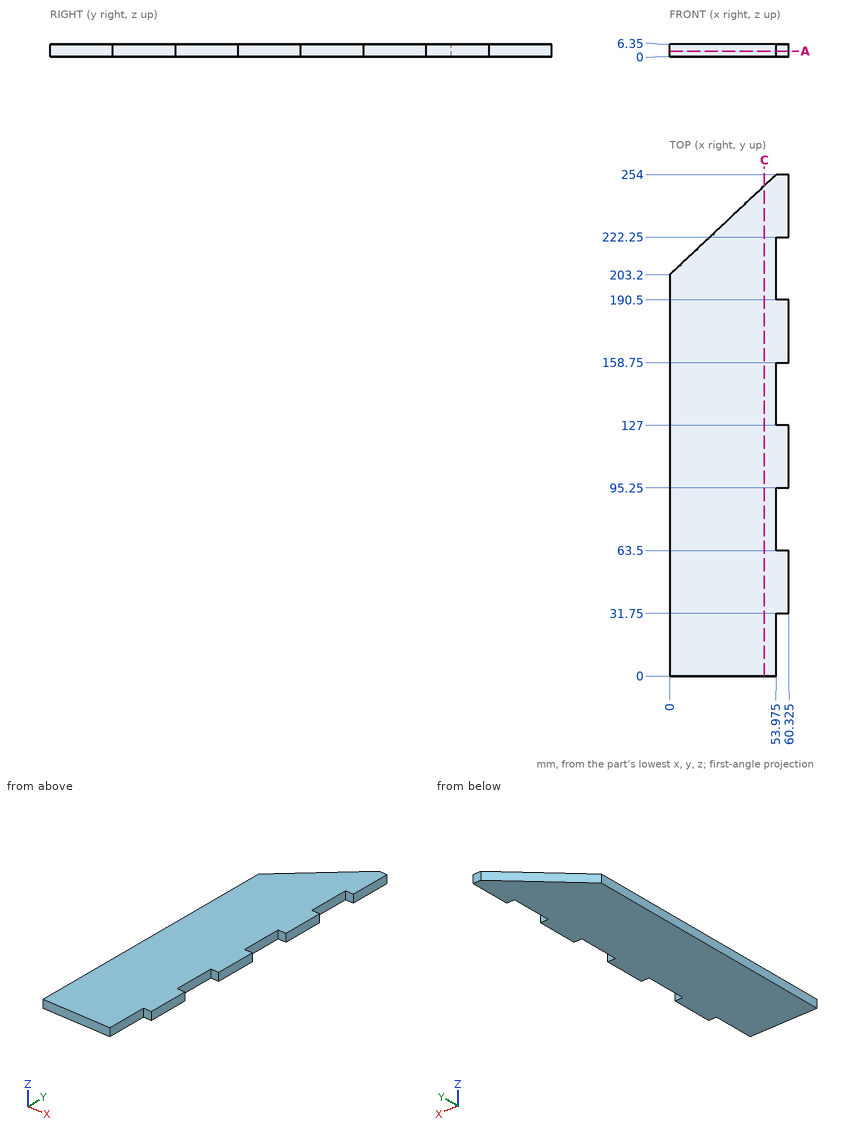
Design review of the part shown in the three views and the two pictorial views. Dimensions are in mm from the part's minimum x, y and z. Give positions to 0.01 mm unless a question says otherwise; leave off trailing zeros. Loops run counter-clockwise (first coordinate to the right, second up) from the corner with the lowest first, then second, coordinate; pieces in that order, holes last. Notation, with made-up numbers: (33, -39.75) -> (45, -39.75) arc R20 ccw to (45, -6.75) -> close; hole circle Ø11 at (51.5, 54.25). An arc over 180 degrees is marked (long way). One line per item, written item: value.
Q1. For pin 1 Ø3 at (x, z) = (56, 3.5) entering from -Y; pin 2 Ø1.9 at (y, z) = (140, 4) entering from +X (3 decimals), all flat-tipped, find the tip position at first contact; note any pin that passes through.
Numbers:
pin 1: stops at y = 31.75
pin 2: stops at x = 53.975
Q2. We need section A-A on z = 2.75. Give the boundary of the cut face in (x, y) (3 decimals), and give its area (3 significant figures).
Numbers:
outline: (0, 0) -> (53.975, 0) -> (53.975, 31.75) -> (60.325, 31.75) -> (60.325, 63.5) -> (53.975, 63.5) -> (53.975, 95.25) -> (60.325, 95.25) -> (60.325, 127) -> (53.975, 127) -> (53.975, 158.75) -> (60.325, 158.75) -> (60.325, 190.5) -> (53.975, 190.5) -> (53.975, 222.25) -> (60.325, 222.25) -> (60.325, 254) -> (53.975, 254) -> (0, 203.2) -> close
area: 13,100 mm^2
Q3. For L1, parallel to Y at x = 56.5, z = 4.5; L2, parallel to X at y = 203, z = 2.25 (3 decimals); L3, parallel to Y at x = 24.5, z = 4.25, list the stretches that pass through material, from the lowest coordinate up.
Numbers:
L1: y = 31.75 to 63.5, 95.25 to 127, 158.75 to 190.5, 222.25 to 254
L2: x = 0 to 53.975
L3: y = 0 to 226.26
Q4. We need section C-C on x = 48. Give the boundary of the cut face in (y, z).
Numbers:
outline: (0, 0) -> (248.38, 0) -> (248.38, 6.35) -> (0, 6.35) -> close
